Verification items for the finished model (mm, model axes). Face numbers are marked on the shaded views. A direction names the side the tool comes from. Round coordinates to 2 decimals unless told otherwise and drop trailing zeros. Order: outer loops, then holes, each group sorted by start corner. A loop starts at its lowest first (then second) coordinate and runs counter-clockwise, first axis right, second up. Notation, with made-up numbers: (-38, -28.75) -> (-3, -28.75) arc R32 ccw to (-3, -1.75) -> close; hole circle Ø9 at (16.25, 64). An arc over 180 degrees is marked (long way). Return JSON: item names as keys, results as strings. Group by question number.
1) Section check C-C on z = 70. Enter the section's corners in (x, y).
2) Section check B-B on x = 0. State how many separate pieces and enclosed holes the cut face has, plus the area to 3 significant figures.
3) Tool access check on the marked faces 4 and 5. Record the directions out of +Z, -Z, +X, -X, +Y, -Y that give a thin tool (end or side, any length) a straight path to the whole face; none if there is none.
4) Scan lines: L1, parallel to Z at x = 29.5, y = -33.5; L2, parallel to Y at x = 0, z = 4.25; L3, parallel to Y at x = 27, z = 14.5. Record each from-to range of solid material in increasing order.
5) Draft check along X on the marked faces 1, 2 and 3. Enter one of: pulls with the +X half, pulls with the -X half, needs draft (parallel to the pull), parting line crosses it, or undercut.
6) Section check D-D on z = 5. Enter the section's corners in (x, y), plus the area to 3 significant figures.
7) Depth check by flat-ended pin: pin 1 (2 mm diameter, centred on y = -36, z = 12.5, fed in from -X); pin 2 (19.5 mm diameter, centred on x = 61.05, y = -35.25, fed in from +Z); pin 3 (5 mm diameter, centred on x = 14, z = 51.5, fed in from +Y). Enter the tip coordinate at first touch or a pass-through.
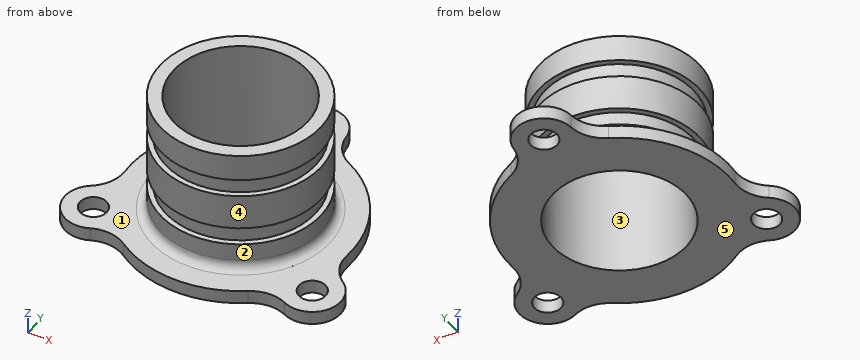
```python
from build123d import *

# Parameters (mm, degrees)
SKETCH_R     = 7.5
PAD_DEPTH    = 7.5
FILLET_R     = 5
SKETCH002_R  = 37.5
POCKET_DEPTH = 77.501


with BuildPart() as part:
    # Sketch → Pad (new body)
    with BuildSketch(Plane.XY):
        with BuildLine():
            ThreePointArc((-27.108608, 55.759514), (-53.693575, 31), (-61.843459, -4.403014))
            ThreePointArc((-70.271756, -22.171485), (-63.722793, -14.394746), (-61.843459, -4.403014))
            ThreePointArc((-70.271756, -22.171485), (-74.911197, -43.25), (-54.336947, -49.771383))
            ThreePointArc((-34.734852, -51.3565), (-44.327612, -47.988185), (-54.336947, -49.771383))
            ThreePointArc((-34.734852, -51.3565), (0, -62), (34.734852, -51.3565))
            ThreePointArc((54.336947, -49.771383), (44.327612, -47.988185), (34.734852, -51.3565))
            ThreePointArc((54.336947, -49.771383), (74.911197, -43.25), (70.271756, -22.171485))
            ThreePointArc((61.843459, -4.403014), (63.722793, -14.394746), (70.271756, -22.171485))
            ThreePointArc((61.843459, -4.403014), (53.693575, 31), (27.108608, 55.759514))
            ThreePointArc((15.934809, 71.942868), (19.395181, 62.38293), (27.108608, 55.759514))
            ThreePointArc((15.934809, 71.942868), (0, 86.5), (-15.934809, 71.942868))
            ThreePointArc((-27.108608, 55.759514), (-19.395181, 62.38293), (-15.934809, 71.942868))
        make_face()
        with Locations((0, 70.5)):
            Circle(SKETCH_R, mode=Mode.SUBTRACT)
        with Locations((-61.054791, -35.25)):
            Circle(SKETCH_R, mode=Mode.SUBTRACT)
        with Locations((61.054791, -35.25)):
            Circle(SKETCH_R, mode=Mode.SUBTRACT)
    extrude(amount=PAD_DEPTH)

    # Sketch001 → Revolution (revolve)
    with BuildSketch(Plane.XZ):
        Polygon((0, 7.5), (45, 7.5), (45, 22.5), (42, 22.5), (42, 32.5), (45, 32.5), (45, 52.5), (42, 52.5), (42, 62.5), (45, 62.5), (45, 77.5), (0, 77.5), align=None)
    revolve(axis=Axis((0, 0, 0), (0, 0, 1)))

    # Fillet
    fillet_edges = [part.edges().sort_by_distance(p)[0] for p in [
        (-45, 0, 7.5),
    ]]
    fillet(fillet_edges, radius=FILLET_R)

    # Sketch002 (on Face28 of Fillet) → Pocket (cut, through all)
    with BuildSketch(Plane.XY.offset(77.5)):
        Circle(SKETCH002_R)
    extrude(amount=-POCKET_DEPTH, mode=Mode.SUBTRACT)


solid = part.part
```
Check result:
{
 "1": {"outline": "circle Ø90 at (0, 0); hole circle Ø75 at (0, 0)"},
 "2": {"separate pieces": "3", "enclosed holes": "0", "area": "1,380 mm^2"},
 "3": {"face 4": "+Z", "face 5": "-Z, +X, -X, +Y, -Y"},
 "4": {"L1": "0 to 22.5, 32.5 to 52.5, 62.5 to 77.5", "L2": "-62 to -37.5, 37.5 to 63, 78 to 86.5", "L3": "-36 to -26.02, 26.02 to 36"},
 "5": {"face 1": "needs draft", "face 2": "parting line crosses it", "face 3": "undercut"},
 "6": {"outline": "(-70.27, -22.17) arc R16 ccw to (-54.34, -49.77) arc R20 cw to (-34.73, -51.36) arc R62 ccw to (34.73, -51.36) arc R20 cw to (54.34, -49.77) arc R16 ccw to (70.27, -22.17) arc R20 cw to (61.84, -4.4) arc R62 ccw to (27.11, 55.76) arc R20 cw to (15.93, 71.94) arc R16 ccw to (-15.93, 71.94) arc R20 cw to (-27.11, 55.76) arc R62 ccw to (-61.84, -4.4) arc R20 cw to start; hole circle Ø15 at (-61.05, -35.25); hole circle Ø75 at (0, 0); hole circle Ø15 at (0, 70.5); hole circle Ø15 at (61.05, -35.25)", "area": "9,400 mm^2"},
 "7": {"pin 1": "x = -28.28", "pin 2": "z = 7.5", "pin 3": "y = 43.51"}
}
